Geometry check sheet. Reference: the model listing, model coordinates, mm. A direction names the side the tool comes from. Give positions to 0.01 mm unless a question says otherwise; leave off trailing zeros. Loops run counter-clockwise (first coordinate to the right, second up) from the corner with the lowest first, then second, coordinate; pieces in that order, holes last.
```python
from build123d import *

# Parameters (mm, degrees)
EXTRUDE_1_DEPTH              = 20
HOLE_WIZARD_M3_1_D           = 2.5
HOLE_WIZARD_M3_1_DEPTH       = 10
HOLE_WIZARD_M3_1_CSINK_D     = 3.05
HOLE_WIZARD_M3_1_CSINK_ANGLE = 90
HOLE_WIZARD_M3_1_TIP         = 0.751075774
HOLE_WIZARD_M3_2_D           = 2.5
HOLE_WIZARD_M3_2_CSINK_D     = 3.05
HOLE_WIZARD_M3_2_CSINK_ANGLE = 90
HOLE_WIZARD_M3_4_D           = 2.5
HOLE_WIZARD_M3_4_CSINK_D     = 3.05
HOLE_WIZARD_M3_4_CSINK_ANGLE = 90
SKETCH_9_W                   = 20
SKETCH_9_H                   = 3.237584756
EXTRUDE_2_DEPTH              = 2
SKETCH_12_W                  = 20
SKETCH_12_H                  = 11.028073375
CUT_EXTRUDE_1_DEPTH          = 39.223029707
SKETCH_13_W                  = 20
SKETCH_13_H                  = 8
EXTRUDE_3_DEPTH              = 2


with BuildPart() as part:
    # 草图1 → 凸台-拉伸1 (new body)
    with BuildSketch(Plane(origin=(0, 0, 0), x_dir=(0, 0, -1), z_dir=(1, 0, 0))):
        Polygon((0, 28), (-2, 28), (-2, -2), (8, -2), (8, 0), (8, 28), align=None)
    extrude(amount=EXTRUDE_1_DEPTH)

    # M3 螺纹孔1
    with Locations(Plane(origin=(5, -2, -3), x_dir=(0, 0, -1), z_dir=(0, -1, 0))):
        with Locations((0, 0), (0, 10)):
            CounterSinkHole(HOLE_WIZARD_M3_1_D / 2, HOLE_WIZARD_M3_1_CSINK_D / 2, depth=HOLE_WIZARD_M3_1_DEPTH, counter_sink_angle=HOLE_WIZARD_M3_1_CSINK_ANGLE)
            with Locations((0, 0, -(HOLE_WIZARD_M3_1_DEPTH + HOLE_WIZARD_M3_1_TIP / 2))):  # 118° drill point
                Cone(0, HOLE_WIZARD_M3_1_D / 2, HOLE_WIZARD_M3_1_TIP, mode=Mode.SUBTRACT)

    # M3 螺纹孔2 (through all)
    with Locations(Plane(origin=(14.7, 14, 2), x_dir=(0, 1, 0), z_dir=(0, 0, 1))):
        with Locations((0, 0), (12, 12)):
            CounterSinkHole(HOLE_WIZARD_M3_2_D / 2, HOLE_WIZARD_M3_2_CSINK_D / 2, counter_sink_angle=HOLE_WIZARD_M3_2_CSINK_ANGLE)

    # M3 螺纹孔4 (through all)
    with Locations(Plane(origin=(5.3, 14, 2), x_dir=(0, 1, 0), z_dir=(0, 0, 1))):
        with Locations((0, 0), (12, -12)):
            CounterSinkHole(HOLE_WIZARD_M3_4_D / 2, HOLE_WIZARD_M3_4_CSINK_D / 2, counter_sink_angle=HOLE_WIZARD_M3_4_CSINK_ANGLE)

    # 草图9 → 凸台-拉伸2 (add)
    with BuildSketch(Plane.XY.offset(2)):
        with Locations((10, 29.381207622)):
            Rectangle(SKETCH_9_W, SKETCH_9_H)
    extrude(amount=-EXTRUDE_2_DEPTH)

    # 草图12 → 切除-拉伸1 (cut, through all)
    with BuildSketch(Plane.XY.offset(2)):
        with Locations((10, 35.514036688)):
            Rectangle(SKETCH_12_W, SKETCH_12_H)
    extrude(amount=-CUT_EXTRUDE_1_DEPTH, mode=Mode.SUBTRACT)

    # 草图13 → 凸台-拉伸3 (add)
    with BuildSketch(Plane(origin=(0, 28, 0), x_dir=(1, 0, 0), z_dir=(0, 1, 0))):
        with Locations((10, 4)):
            Rectangle(SKETCH_13_W, SKETCH_13_H)
    extrude(amount=EXTRUDE_3_DEPTH)


solid = part.part
```
1) Depth check by flat-ended pin: P1, Ø2, axis at x = 15, z = -3, coming from the -Y side; P2, Ø1.5, axis at x = 5, z = -3, coming from the -Y side; P3, Ø3, axis at x = 5.3, y = 14, coming from the +Z side (3 decimals); P4, Ø2, axis at x = 2.7, y = 26, coming from the +Z side. Enter the tip coordinate at first touch or a pass-through.
2) Mould release check, pull along Z, two halves, no side actions. Record for faces 3 (the flat face through (10, 14, 2)), 4 (the cylindrical face through (3.891, 3.206, -2.423)), 5 (the flat face through (10, -2, -3)): +Z half, -Z half, draft (parallel to the pull), parting line (faces both ways), or undercut.
3) Sectioned sample at B-B on x = 2.7. Enter the section's corners in (y, z) (3 decimals), plus the area to 3 significant figures.
4) Scan lines: line 1 along X through (y, z) = (26, -4); line 2 along X through (y, z) = (14, -1.25); line 3 along Y through (x, z) = (17.3, -1). Record each from-to range of solid material in increasing order.
5) Tool access check on faces 1 (the cylindrical face through (16.054, 3.206, -2.328)), 2 (the flat face through (0, 14, -3)). Record the directions out of +Z, -Z, +X, -X, +Y, -Y that give a thin tool (end or side, any length) a straight path to the whole face; none if there is none.
6) Sectioned sample at C-C on z = -6.5. Enter the section's corners in (x, y), plus the area to 3 significant figures.
7) Sectioned sample at A-A on y = 26. Enter the section's corners in (x, z) (3 decimals), plus the area to 3 significant figures.
Determined:
1. P1: stops at y = 8.15
1. P2: stops at y = 8.3
1. P3: stops at z = 1.975
1. P4: passes through
2. face 3: +Z half
2. face 4: undercut
2. face 5: draft
3. outline: (-2, -8) - (24.75, -8) - (24.75, 1.725) - (24.475, 2) - (-2, 2) - close; (27.25, -8) - (30, -8) - (30, 2) - (27.525, 2) - (27.25, 1.725) - close
3. area: 295 mm2
4. line 1: x = 0 to 1.45, 3.95 to 16.05, 18.55 to 20
4. line 2: x = 0 to 4.05, 6.55 to 13.45, 15.95 to 20
4. line 3: y = -2 to 24.75, 27.25 to 30
5. face 1: -Y
5. face 2: +Z, -Z, -X, +Y, -Y
6. outline: (0, -2) - (20, -2) - (20, 30) - (0, 30) - close; hole circle Ø2.5 at (2.7, 26); hole circle Ø2.5 at (5.3, 14); hole circle Ø2.5 at (14.7, 14); hole circle Ø2.5 at (17.3, 26)
6. area: 620 mm2
7. outline: (0, -8) - (1.45, -8) - (1.45, 1.725) - (1.175, 2) - (0, 2) - close; (3.95, -8) - (16.05, -8) - (16.05, 1.725) - (15.775, 2) - (4.225, 2) - (3.95, 1.725) - close; (18.55, -8) - (20, -8) - (20, 2) - (18.825, 2) - (18.55, 1.725) - close
7. area: 150 mm2
